For this review, take the finished solid that the model builds, in its own axes (mm). A direction names the side the tool comes from. Coordinates: 2 decimals unless noted, no trailing zeros. Loops run counter-clockwise (first coordinate to the right, second up) from the corner with the lowest first, then second, coordinate; pieces in that order, holes last. Notation, with made-up numbers: (76, 89.5) -> (114, 89.5) arc R16 cw to (114, 105.5) -> close; hole circle Ø4 at (74, 61.5). An arc over 180 degrees is marked (long way). Answer in a Markdown table with one row per item.
from build123d import *

# Parameters (mm, degrees)
F0_R     = 11
F0_R_2   = 5
F1_DEPTH = 1
F2_SIZE  = 0.5
F0_R_3   = 4.05
F3_DEPTH = 1.8
F4_DEPTH = 5.2
F5_R     = 0.5
F6_SIZE  = 0.5


with BuildPart() as f1:
    # F0 (on Top) → F1 (new body)
    with BuildSketch(Plane.XY):
        Circle(F0_R)
        Circle(F0_R_2, mode=Mode.SUBTRACT)
    extrude(amount=F1_DEPTH)

    # F2
    f2_edges = [f1.edges().sort_by_distance(p)[0] for p in [
        (-11, 0, 1),
    ]]
    chamfer(f2_edges, length=F2_SIZE)

    # F0 (on Top) → F3 (join)
    with BuildSketch(Plane.XY):
        Circle(F0_R_2)
        Circle(F0_R_3, mode=Mode.SUBTRACT)
    extrude(amount=F3_DEPTH)

    # F0 (on Top) → F4 (join)
    with BuildSketch(Plane.XY):
        Circle(F0_R_3)
    extrude(amount=F4_DEPTH)

    # F5
    f5_edges = [f1.edges().sort_by_distance(p)[0] for p in [
        (-4.05, 0, 5.2),
    ]]
    fillet(f5_edges, radius=F5_R)

    # F6
    f6_edges = [f1.edges().sort_by_distance(p)[0] for p in [
        (-5, 0, 1.8),
    ]]
    chamfer(f6_edges, length=F6_SIZE)


solid = f1.part
Item 1: Take a section at A-A, the plane x = 0. State the section outline as (y, z) points, and give its area (3 significant figures).
Worked answers:
| item | result |
|---|---|
| outline | (-11, 0) -> (11, 0) -> (11, 0.5) -> (10.5, 1) -> (5, 1) -> (5, 1.3) -> (4.5, 1.8) -> (4.05, 1.8) -> (4.05, 4.7) arc R0.5 ccw to (3.55, 5.2) -> (-3.55, 5.2) arc R0.5 ccw to (-4.05, 4.7) -> (-4.05, 1.8) -> (-4.5, 1.8) -> (-5, 1.3) -> (-5, 1) -> (-10.5, 1) -> (-11, 0.5) -> close |
| area | 56.9 mm² |
Item 2: Insertion check: pin 1 (1 mm diameter, centred on x = -1, z = 2.5, fed in from +Y); pin 2 (1.5 mm diameter, centred on x = 6.5, y = -1.5, fed in from +Z); pin 3 (1.5 mm diameter, centred on y = 8, z = 1.5, fed in from -X). Each pin has a flat end and moves straight along its axis. Give the tip position at first contact, or say it passes through.
Worked answers:
| item | result |
|---|---|
| pin 1 | y = 4.02 |
| pin 2 | z = 1 |
| pin 3 | x = -7.44 |
Item 3: For L1, parallel to Z at x = -2.75, y = -6.5; L2, parallel to Y at x = -3.5, z = 1.7; L3, parallel to Y at x = 0.75, z = 3.65, list the stretches that pass through material, from the lowest coordinate up.
Worked answers:
| item | result |
|---|---|
| L1 | 0 to 1 |
| L2 | -2.98 to 2.98 |
| L3 | -3.98 to 3.98 |
Item 4: Take a section at C-C, the plane z = 3. State the section outline as (x, y) points.
Worked answers:
| item | result |
|---|---|
| outline | circle Ø8.1 at (0, 0) |
Item 5: For faces 1 (the cylindrical face through (-2.38, -10.74, 0.25)), 2 (the cylindrical face through (-0.878, -3.954, 3.23)), list the 3-axis set-ups (+Z, -Z, +X, -X, +Y, -Y) from which the entire face can be reached by the end or side of a thin tool; tool diameter is ignored.
Worked answers:
| item | result |
|---|---|
| face 1 | +Z, -Z |
| face 2 | +Z |
